```python
from build123d import *

# Parameters (mm, degrees)
SKETCH1_R           = 57.5
SKETCH1_R_2         = 25
BOSS_EXTRUDE1_DEPTH = 16
CHAMFER1_SIZE       = 2
CHAMFER2_SIZE       = 10


with BuildPart() as part:
    # Sketch1 → Boss-Extrude1 (new, symmetric)
    with BuildSketch(Plane.XY):
        Circle(SKETCH1_R)
        Circle(SKETCH1_R_2, mode=Mode.SUBTRACT)
    extrude(amount=BOSS_EXTRUDE1_DEPTH, both=True)

    # Chamfer1
    chamfer1_edges = [part.edges().sort_by_distance(p)[0] for p in [
        (-57.5, 0, -16),
        (-57.5, 0, 16),
    ]]
    chamfer(chamfer1_edges, length=CHAMFER1_SIZE)

    # Chamfer2
    chamfer2_edges = [part.edges().sort_by_distance(p)[0] for p in [
        (-25, 0, 16),
    ]]
    chamfer(chamfer2_edges, length=CHAMFER2_SIZE)


solid = part.part
```
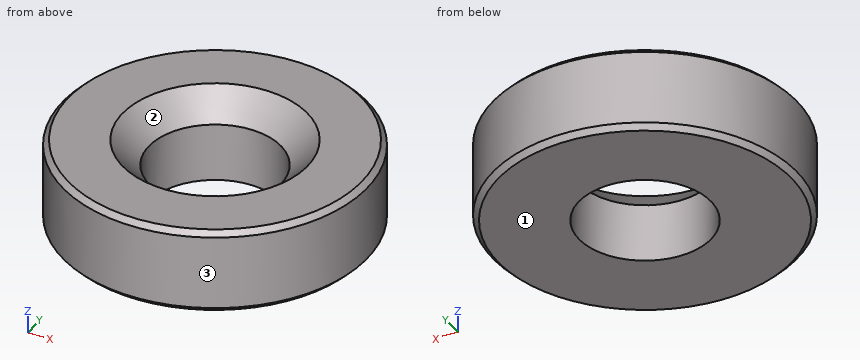
Part model, mm, in its own coordinate system. Face numbers are marked on the shaded views. Round coordinates to 2 decimals unless told otherwise and drop trailing zeros. Write each loop counter-clockwise with the first axis right and the second up, starting at its lowest first coordinate (ties: lowest second). Pieces come first, ordered by that corner, then holes. Notation, with made-up numbers: M -12,87.25 L 7,87.25 A12 ccw 7,97.25 Z; hole C 87,5.25 d4. An arc over 180 degrees is marked long. One line per question, with ' | ' between items.
(1) Pin check, flat tips, straight feed: pin 1 (1.5 mm diameter, centred on x = -40, z = -1, fed in from +Y); pin 2 (4 mm diameter, centred on x = -28, z = 12, fed in from -Y); pin 3 (1 mm diameter, centred on x = -40, z = 1.5, fed in from +Y). Stop position of each tip, or through.
Answer key:
pin 1: stops at y = 42.02 | pin 2: stops at y = -51.29 | pin 3: stops at y = 41.79
(2) Saw through at A-A on x = 0. Write the cut outline in (y, z), then the cut area to 3 significant figures.
Answer key:
outline: M -57.5,-14 L -55.5,-16 L -25,-16 L -25,6 L -35,16 L -55.5,16 L -57.5,14 Z; M 25,-16 L 55.5,-16 L 57.5,-14 L 57.5,14 L 55.5,16 L 35,16 L 25,6 Z | area: 1,970 mm^2
(3) Probe line 1 along Y through (x, z) = (0, -10); line 2 along Y through (x, z) = (-10, -5); line 3 along X through (y, z) = (-17, 4). List the from-to ranges inside material, lowest first.
Answer key:
line 1: y = -57.5 to -25, 25 to 57.5 | line 2: y = -56.62 to -22.91, 22.91 to 56.62 | line 3: x = -54.93 to -18.33, 18.33 to 54.93
(4) Saw through at C-C on z = 7.5. Write the cut outline in (x, y).
Answer key:
outline: C 0,0 d115; hole C 0,0 d53
(5) Two-plate mould, pull along Z, no slides. Class the marked faces 1, 2 and 3: released by +Z, released by -Z, zero draft, split by the parting line, or undercut.
Answer key:
face 1: released by -Z | face 2: released by +Z | face 3: zero draft
(6) Saw through at D-D on z = -1. Write the cut outline in (x, y), then the cut area to 3 significant figures.
Answer key:
outline: C 0,0 d115; hole C 0,0 d50 | area: 8,420 mm^2
